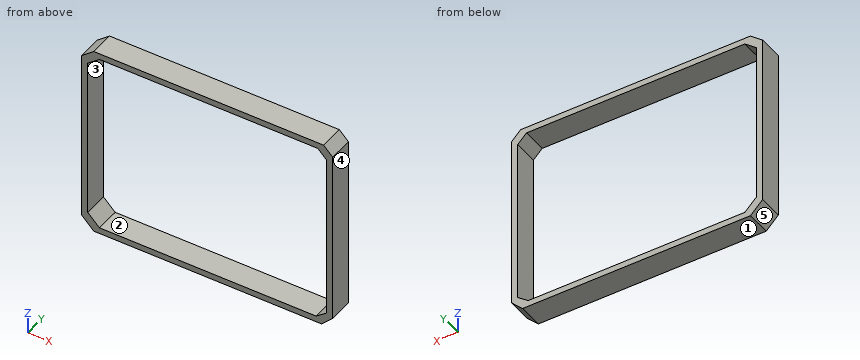
Autodesk Inventor part; units mm, degrees
ref_plane "YZ Plane" through (0, 0, 0) normal (1, 0, 0) x (0, 1, 0)
ref_plane "XZ Plane" through (0, 0, 0) normal (0, 1, 0) x (-1, 0, 0)
ref_plane "XY Plane" through (0, 0, 0) normal (0, 0, 1) x (1, 0, 0)
sketch "Sketch1" plane through (0, 0, 0) normal (0, 1, 0) x (-1, 0, 0)
  line L0 (-35.1948, -29.8974) -> (39.3106, -29.8974)
  line L1 (43.2831, -25.9239) -> (39.3106, -29.8974)
  line L2 (-35.1948, -29.8974) -> (39.3106, -29.8974)
  line L3 (39.3106, -29.8974) -> (43.2831, -25.9239)
  line L4 (43.2831, -25.9239) -> (43.2831, 30.6268)
  line L5 (43.2831, 30.6268) -> (39.3102, 33.8564)
  line L6 (39.3102, 33.8564) -> (-35.8021, 33.8465)
  line L7 (-38.7786, 22.9053) -> (-38.7786, 30.8692)
  line L8 (-35.8021, 33.8465) -> (-38.7786, 30.8692)
  line L9 (-38.7786, 30.8692) -> (-38.7786, -26.3136)
  line L10 (-38.7786, -26.3136) -> (-35.1948, -29.8974)
  line L11 (-35.1948, -29.8974) -> (-38.7786, -26.3136)
  line L12 (-33.3338, -27.8974) -> (37.4464, -27.8974)
  line L13 (41.2831, -24.1074) -> (37.4464, -27.8974)
  line L14 (-33.3338, -27.8974) -> (37.4464, -27.8974)
  line L15 (37.4464, -27.8974) -> (41.2831, -24.1074)
  line L16 (41.2831, -24.1074) -> (41.2831, 28.8221)
  line L17 (41.2831, 28.8221) -> (37.4463, 31.8562)
  line L18 (37.4463, 31.8562) -> (-33.9105, 31.8467)
  line L19 (-36.7786, 21.447) -> (-36.7786, 29.0134)
  line L20 (-33.9105, 31.8467) -> (-36.7786, 29.0134)
  line L21 (-36.7786, 29.0134) -> (-36.7786, -25.3109)
  line L22 (-36.7786, -25.3109) -> (-33.3338, -27.8974)
  line L23 (-33.3338, -27.8974) -> (-36.7786, -25.3109)
  dimension "d1" = 2
  dimension "d2" = 2
  dimension "d3" = 2
  dimension "d4" = 2
extrude "Extrusion1" add sketch "Sketch1" along normal blind 8
properties part number "Mash Tank Bottom"
Can you work these out from the model? Positions are in its coordinate system, mm. Face numbers are marked on the shaded views. A direction names the side the tool comes from. Give positions to 0.01 mm unless a question says otherwise; leave off trailing zeros. Loops run counter-clockwise (first coordinate to the right, second up) from the corner with the lowest first, then second, coordinate; pieces in that order, holes last. Notation, with made-up numbers: M 57,-26 L 106,-26 A19 cw 106,-9 Z; hole C -9.5,24 d6. An arc over 180 degrees is marked long. One line per question, with ' | ' between items. Start each with the question number.
Q1. For the marked faces 1 and 2, which set-ups out of +Z, -Z, +X, -X, +Y, -Y let a thin tool reach every point of the face, with its end or its side?
Q2. If we mould it in two halves opening along Z, with no side actions, what happens to the marked faces 3, 4 and 5? For each: +Z half, -Z half, draft (parallel to the pull), parting line (faces both ways), or undercut.
Q3. If I drill on line 1 (Z direction, x = -6, y = 2.5); line 2 (X direction, y = 1, z = -24), over which ranges is the centre line in solid material (lowest first)? Write a range as from..to.
Q4. If we section it at A-A (z = 8): Please give me the cut outline in (x, y), plus the area to 3 significant figures.
Q5. If we section it at B-B (x = 8.5): Please give me the cut outline in (y, z).
Q6. If we section it at C-C (y = 6.5): Please give me the cut outline in (x, z), plus the area to 3 significant figures.
Q7. For pin 1 Ø2.5 at (x, y) = (-19, 5) entering from +Z, with a flat end and sliding along its axis, tell me the tip position at first contact or that it passes through.
Computed:
1) face 1: -Z, +X, -X, +Y, -Y | face 2: +Y, -Y
2) face 3: undercut | face 4: draft | face 5: -Z half
3) line 1: z = -29.9..-27.9, 31.85..33.85 | line 2: x = -43.28..-41.28, 36.78..38.78
4) outline: M -43.28,0 L -41.28,0 L -41.28,8 L -43.28,8 Z; M 36.78,0 L 38.78,0 L 38.78,8 L 36.78,8 Z | area: 32.0 mm²
5) outline: M 0,-29.9 L 8,-29.9 L 8,-27.9 L 0,-27.9 Z; M 0,31.85 L 8,31.85 L 8,33.85 L 0,33.85 Z
6) outline: M -43.28,-25.92 L -39.31,-29.9 L 35.19,-29.9 L 38.78,-26.31 L 38.78,30.87 L 35.8,33.85 L -39.31,33.86 L -43.28,30.63 Z; hole M -41.28,-24.11 L -37.45,-27.9 L 33.33,-27.9 L 36.78,-25.31 L 36.78,29.01 L 33.91,31.85 L -37.45,31.86 L -41.28,28.82 Z | area: 564 mm²
7) pin 1: stops at z = 33.85
